Work out the finished part from the listing and answer in its coordinate system (mm). A direction names the side the tool comes from. Give positions to 0.01 mm unless a question says otherwise; leave off trailing zeros. Order: outer loops, then holes, each group sorted by start corner. A loop starts at its lowest first (then second) coordinate and runs counter-clockwise, first axis right, second up. Notation, with made-up numbers: M -33.5,-19 L -23.5,-19 A25 ccw -23.5,15 Z; hole C 25.5,5.5 d9. An arc over 180 degrees is marked long. One line per item, written item: value.
from build123d import *

# Parameters (mm, degrees)
SKETCH1_W           = 100
SKETCH1_H           = 63
BOSS_EXTRUDE1_DEPTH = 12
SKETCH2_R           = 25
BOSS_EXTRUDE2_DEPTH = 50
BOSS_EXTRUDE3_DEPTH = 10
RIB1_REACH          = 142.335
SKETCH4_WALL_W      = 337.241680066
SKETCH4_WALL_H      = 10
BOSS_EXTRUDE4_START = 3
SKETCH5_W           = 32
SKETCH5_H           = 32
BOSS_EXTRUDE4_DEPTH = 12
BOSS_EXTRUDE5_START = 3
SKETCH5_2_W         = 32
SKETCH5_2_H         = 32
BOSS_EXTRUDE5_DEPTH = 12
SKETCH6_W           = 3
SKETCH6_H           = 46.09785454
CUT_EXTRUDE1_DEPTH  = 157.843871414
HOLE1_D             = 25
HOLE2_D             = 12
HOLE3_D             = 14
HOLE3_DEPTH         = 12
FILLET1_R           = 25


with BuildPart() as part:
    # Sketch1 → Boss-Extrude1 (new body)
    with BuildSketch(Plane(origin=(0, 0, 0), x_dir=(1, 0, 0), z_dir=(0, 1, 0))):
        with Locations((0, 31.5)):
            Rectangle(SKETCH1_W, SKETCH1_H)
    extrude(amount=BOSS_EXTRUDE1_DEPTH)



with BuildPart() as body_2:
    # Sketch2 → Boss-Extrude2 (new body)
    with BuildSketch(Plane.XY):
        with Locations((0, 90)):
            Circle(SKETCH2_R)
    extrude(amount=-BOSS_EXTRUDE2_DEPTH)


with BuildPart() as part_1:
    add(part.part)

    add(body_2.part)  # Boss-Extrude3 merges body 2
    # Sketch3 → Boss-Extrude3 (add)
    with BuildSketch(Plane.XY):
        with BuildLine():
            Line((-50, 12), (50, 12))
            Line((50, 12), (23.906779363, 97.312038053))
            ThreePointArc((23.906779363, 97.312038053), (0, 115), (-23.906779363, 97.312038053))
            Line((-23.906779363, 97.312038053), (-50, 12))
        make_face()
    extrude(amount=-BOSS_EXTRUDE3_DEPTH)

    # Sketch4 wall → Rib1 (add, up to next)
    with BuildSketch(Plane(origin=(0, 38.5, -56.5), x_dir=(0, 0.971210844098, 0.238221527798), z_dir=(0, -0.238221527798, 0.971210844098)), mode=Mode.PRIVATE) as rib1_sk1:
        Rectangle(SKETCH4_WALL_W, SKETCH4_WALL_H)
    rib1_tool1 = extrude(rib1_sk1.sketch, amount=RIB1_REACH, mode=Mode.PRIVATE) - part_1.part
    add(rib1_tool1.solids().sort_by_distance((0, 38.5, -56.5))[0])



with BuildPart() as body_2_2:
    # Sketch5 → Boss-Extrude4 (new body)
    with BuildSketch(Plane(origin=(0, 0, 0), x_dir=(0, 0, -1), z_dir=(1, 0, 0)).offset(BOSS_EXTRUDE4_START)):
        with Locations((22, 124)):
            Rectangle(SKETCH5_W, SKETCH5_H)
    extrude(amount=BOSS_EXTRUDE4_DEPTH)


with BuildPart() as part_2:
    add(part_1.part)

    add(body_2_2.part)  # Boss-Extrude5 merges body 2 2
    # Sketch5<2> → Boss-Extrude5 (add)
    with BuildSketch(Plane(origin=(0, 0, 0), x_dir=(0, 0, -1), z_dir=(1, 0, 0)).offset(BOSS_EXTRUDE5_START)):
        with Locations((22, 124)):
            Rectangle(SKETCH5_2_W, SKETCH5_2_H)
    boss_extrude5 = extrude(amount=BOSS_EXTRUDE5_DEPTH)

    # Mirror7: Boss-Extrude5 across plane
    add(boss_extrude5.mirror(Plane(origin=(0, 0, 0), x_dir=(0, 0, 1), z_dir=(1, 0, 0))))

    # Sketch6 → Cut-Extrude1 (cut, through all)
    with BuildSketch(Plane(origin=(0, 0, -50), x_dir=(-1, 0, 0), z_dir=(0, 0, -1))):
        with Locations((0, 116.95107273)):
            Rectangle(SKETCH6_W, SKETCH6_H)
    extrude(amount=-CUT_EXTRUDE1_DEPTH, mode=Mode.SUBTRACT)

    # Hole1 (through all)
    with Locations(Plane(origin=(0, 0, -50), x_dir=(-1, 0, 0), z_dir=(0, 0, -1))):
        with Locations((0, 90)):
            Hole(HOLE1_D / 2)

    # Hole2 (through all)
    with Locations(Plane.ZY.offset(15)):
        with Locations((-22, 128)):
            Hole(HOLE2_D / 2)

    # Hole3
    with Locations(Plane(origin=(0, 12, 0), x_dir=(1, 0, 0), z_dir=(0, 1, 0))):
        with Locations((-25, 38), (25, 38)):
            Hole(HOLE3_D / 2, depth=HOLE3_DEPTH)

    # Fillet1
    fillet1_edges = [part_2.edges().sort_by_distance(p)[0] for p in [
        (-50, 6, -63),
        (50, 6, -63),
    ]]
    fillet(fillet1_edges, radius=FILLET1_R)


solid = part_2.part
(1) Section D-D, the plane z = -14.5 is taken. Give the vertices of the cut face in (x, y).
Findings:
outline: M -50,0 L 50,0 L 50,12 L 5,12 L 5,65.51 A25 ccw 15,110 L 15,140 L 3,140 L 3,114.82 A25 ccw 1.5,114.95 L 1.5,102.41 A12.5 cw long -1.5,102.41 L -1.5,114.95 A25 ccw -3,114.82 L -3,140 L -15,140 L -15,110 A25 ccw -5,65.51 L -5,12 L -50,12 Z
(2) Section C-C, the plane x = -9.5 is taken. Give the vertices of the cut face in (y, z).
Findings:
outline: M 0,-63 L 12,-63 L 12,-10 L 66.88,-10 L 66.88,-50 L 81.88,-50 L 81.88,0 L 0,0 Z; M 98.12,-50 L 113.12,-50 L 113.12,-38 L 140,-38 L 140,-6 L 113.12,-6 L 113.12,0 L 98.12,0 Z; hole C 128,-22 d12
(3) Section B-B, the plane y = 128 is taken. Give the vertices of the cut face in (x, z), then the cut area to 3 significant figures.
Findings:
outline: M -15,-38 L -3,-38 L -3,-28 L -15,-28 Z; M -15,-16 L -3,-16 L -3,-6 L -15,-6 Z; M 3,-38 L 15,-38 L 15,-28 L 3,-28 Z; M 3,-16 L 15,-16 L 15,-6 L 3,-6 Z
area: 480 mm^2
(4) Section A-A, the plane z = -22 is taken. Give the vertices of the cut face in (x, y), then the cut area to 3 significant figures.
Findings:
outline: M -50,0 L 50,0 L 50,12 L 5,12 L 5,65.51 A25 ccw 15,110 L 15,122 L 3,122 L 3,114.82 A25 ccw 1.5,114.95 L 1.5,102.41 A12.5 cw long -1.5,102.41 L -1.5,114.95 A25 ccw -3,114.82 L -3,122 L -15,122 L -15,110 A25 ccw -5,65.51 L -5,12 L -50,12 Z; M -15,134 L -3,134 L -3,140 L -15,140 Z; M 3,134 L 15,134 L 15,140 L 3,140 Z
area: 3,530 mm^2
(5) Find the intervals of material crossed by probe 1 along X at (y, z) = (7, -38); probe 2 along Y at (x, z) = (-11.5, -17); probe 3 along X at (y, z) = (90, -10.5), in increasing order. Write a range as from..to.
Findings:
probe 1: x = -50..-32, -18..18, 32..50
probe 2: y = 0..12, 67.8..85.1, 94.9..124.68, 131.32..140
probe 3: x = -25..-12.5, 12.5..25
(6) Determine the mould class of faces 5 (the flat face through (-1, 0, -32)), 6 (the cylindrical face through (42.871, 6.084, -55.482)), 7 (the cylindrical face through (-0.53, 77.51, -24.65)) for opening direction Y: pulls with the +Y half, pulls with the -Y half, needs draft (parallel to the pull), parting line crosses it, or undercut.
Findings:
face 5: pulls with the -Y half
face 6: needs draft
face 7: undercut
(7) Which of the six approach directions +Z, -Z, +X, -X, +Y, -Y give full straight-line access (tool end or side, diameter ignored) to faces 1 (the cylindrical face through (25.91, 5.92, -44.94)), 2 (the flat face through (-5, 37, -31)), 3 (the flat face through (22, 46, -10)), 4 (the flat face through (-15, 122, -25))?
Findings:
face 1: -Y
face 2: -Z, -X
face 3: -Z, +X
face 4: +Z, -Z, -X, +Y
(8) Given P1, Ø1.5, axis at x = 11.5, y = 123, coming from the +Z side; P2, Ø4, axis at y = 64.5, z = -6.5, coming from the +X side; P3, Ø15, axis at y = 126.5, z = -17, coming from the +X side; P4, Ø7, axis at y = 128, z = -22, coming from the -X side, each flat-ended and moving along its own axis, determine where each tip first touches the part or whether it passes through.
Findings:
P1: stops at z = -6
P2: stops at x = 34.55
P3: stops at x = 15
P4: passes through
